Geometry: final body of the model. Coordinates: model frame, mm. Face numbers are marked on the shaded views. A direction names the side the tool comes from. Give positions to 0.01 mm unless a question says otherwise; leave off trailing zeros. Loops run counter-clockwise (first coordinate to the right, second up) from the corner with the lowest first, then second, coordinate; pieces in that order, holes last. Notation, with made-up numbers: (2.5, 11.5) -> (13.5, 11.5) arc R16 ccw to (13.5, 20.5) -> close; hole circle Ø6 at (-19, -19). An arc over 180 degrees is marked (long way). Answer in a Markdown table with one row per item. Add a question column.
1) Section query A-A (x = 0). Return the cut outline in (y, z).
2) Section query C-C (z = 246). Return the cut outline in (x, y), plus the area to 3 significant figures.
3) First-contact query: P1, Ø10, axis at x = 4, y = -26, coming from the +Z side; P2, Ø1.5, axis at y = 17, z = -148.5, coming from the -X side; P3, Ø3, axis at y = -14.5, z = -160, coming from the -X side. Flat tips, straight axial feed; report the tip coordinate or a pass-through.
4) Section query D-D (y = -28). Return the cut outline in (x, z), plus the area to 3 significant figures.
5) Access query for the marked faces 1, 2 and 3. Directions: +Z, -Z, +X, -X, +Y, -Y. A direction counts if a zero-diameter tool reaches every point of the face in a straight line with its end or side. Return the directions, or none.
6) Line query: line 1 (Y direction, x = 3, z = 50); line 2 (Z direction, x = 10, y = -22.5); line 3 (Y direction, x = 0, z = 142). Output: solid intervals per line, ascending. Write a range as from..to.
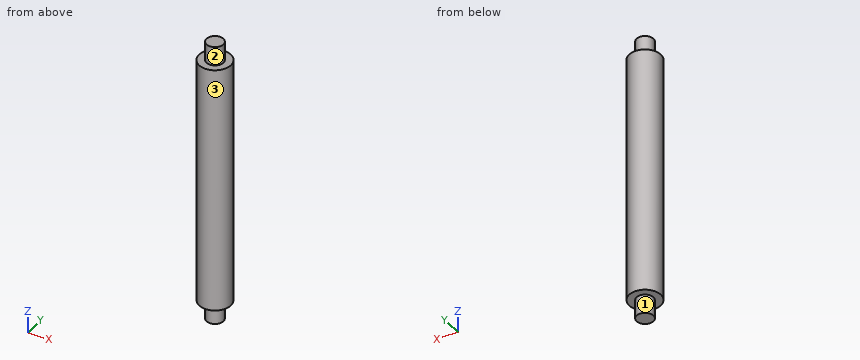
```python
from build123d import *

# Parameters (mm, degrees)
SKETCH1_R           = 37.5
BOSS_EXTRUDE1_DEPTH = 295
SKETCH2_R           = 20
BOSS_EXTRUDE2_DEPTH = 45
BOSS_EXTRUDE3_START = 45
SKETCH3_R           = 20
BOSS_EXTRUDE3_DEPTH = 45


with BuildPart() as part:
    # Sketch1 → Boss-Extrude1 (new, symmetric)
    with BuildSketch(Plane.XY):
        Circle(SKETCH1_R)
    extrude(amount=BOSS_EXTRUDE1_DEPTH, both=True)

    # Sketch2 → Boss-Extrude2 (add)
    with BuildSketch(Plane.XY.offset(295)):
        with Locations(Location((0, 0, 0), (0, 0, 180))):
            Circle(SKETCH2_R)
    extrude(amount=BOSS_EXTRUDE2_DEPTH)

    # Sketch3 → Boss-Extrude3 (add)
    with BuildSketch(Plane(origin=(0, 0, -295), x_dir=(-1, 0, 0), z_dir=(0, 0, -1)).offset(BOSS_EXTRUDE3_START)):
        Circle(SKETCH3_R)
    extrude(amount=-BOSS_EXTRUDE3_DEPTH)


solid = part.part
```
Evaluation:
| question | item | result |
|---|---|---|
| 1 | outline | (-37.5, -295) -> (-20, -295) -> (-20, -340) -> (20, -340) -> (20, -295) -> (37.5, -295) -> (37.5, 295) -> (20, 295) -> (20, 340) -> (-20, 340) -> (-20, 295) -> (-37.5, 295) -> close |
| 2 | outline | circle Ø75 at (0, 0) |
| 2 | area | 4,420 mm² |
| 3 | P1 | z = 295 |
| 3 | P2 | x = -33.8 |
| 3 | P3 | x = -35.17 |
| 4 | outline | (-24.94, -295) -> (24.94, -295) -> (24.94, 295) -> (-24.94, 295) -> close |
| 4 | area | 29,400 mm² |
| 5 | face 1 | -Z |
| 5 | face 2 | +Z |
| 5 | face 3 | +Z, -Z |
| 6 | line 1 | -37.38..37.38 |
| 6 | line 2 | -295..295 |
| 6 | line 3 | -37.5..37.5 |
